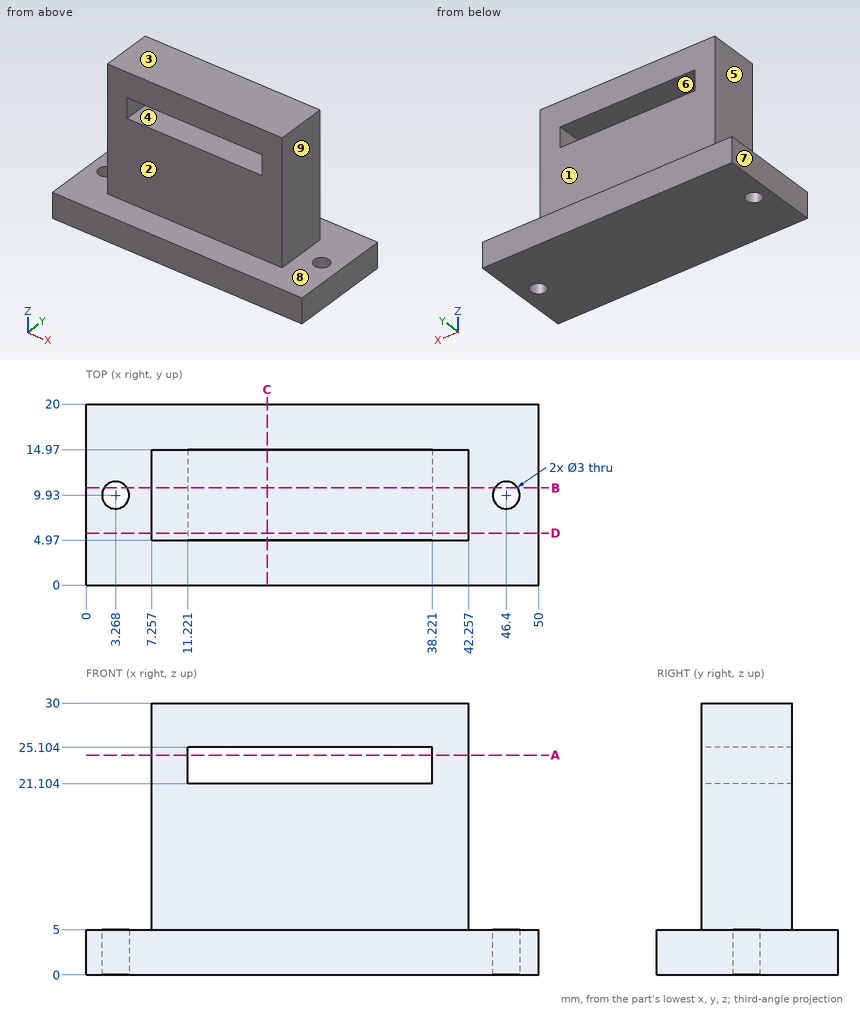
Print and shaded views of the part. All mm, measured from the part's lowest x, y and z. A direction names the side the tool comes from. Round coordinates to 2 decimals unless told otherwise and drop trailing zeros. Write each loop counter-clockwise with the first axis right and the second up, starting at its lowest first coordinate (ties: lowest second). Pieces come first, ordered by that corner, then holes. Notation, with made-up numbers: (75, -22) -> (99, -22) arc R6 ccw to (99, -15) -> close; hole circle Ø5 at (-15.75, -37). An arc over 180 degrees is marked (long way). Answer in a Markdown table with one row per item. Add a question column.
Item 1: Which spindle directions (+Z, -Z, +X, -X, +Y, -Y) get a long thin tool onto all of the face, cutting with end or side? Do the marked faces 1, 2, 3, 4 and 5. Say none if no direction does.
Item 2: Saw through at A-A, the plane z = 24.25. Write the cut outline in (x, y), then the cut area to 3 significant figures.
Item 3: Saw through at D-D, the plane y = 5.75. Write the cut outline in (x, z) (1 decimal), then the cut area to 3 significant figures.
Item 4: Mould opens along X. For the marked faces 6, 7, 8 and 9 say: pulls with the +X half, pulls with the -X half, needs draft (parallel to the pull), parting line crosses it, or undercut.
Item 5: Saw through at B-B, the plane y = 10.75. Write the cut outline in (x, z) (1 decimal), then the cut area to 3 significant figures.
Item 6: Saw through at C-C, the plane x = 20. Write the cut outline in (y, z) (1 decimal).
Item 7: Drop flat-ended pins along their axis: pin 1 Ø2 at (y, z) = (8, 19) entering from -X; pin 2 Ø5 at (y, z) = (7.5, 14.5) entering from +X; pin 3 Ø1.5 at (x, y) = (39.5, 4) entering from +Z. Give the stop position or say it passes through.
Item 8: Drill centre lines: line 1 (Z direction, x = 13, y = 7.25) (1 decimal); line 2 (Y direction, x = 35, z = 27.75); line 3 (Z direction, x = 20, y = 3.5). Where is each one in solid material? Low to high. Write a range as from..to.
Findings below:
| question | item | result |
|---|---|---|
| 1 | face 1 | +Z, +X, -X, +Y |
| 1 | face 2 | +Z, +X, -X, -Y |
| 1 | face 3 | +Z, +X, -X, +Y, -Y |
| 1 | face 4 | +Y, -Y |
| 1 | face 5 | +Z, -X, +Y, -Y |
| 2 | outline | (7.26, 4.97) -> (11.22, 4.97) -> (11.22, 14.97) -> (7.26, 14.97) -> close; (38.22, 4.97) -> (42.26, 4.97) -> (42.26, 14.97) -> (38.22, 14.97) -> close |
| 2 | area | 80.0 mm^2 |
| 3 | outline | (0, 0) -> (50, 0) -> (50, 5) -> (42.3, 5) -> (42.3, 30) -> (7.3, 30) -> (7.3, 5) -> (0, 5) -> close; hole (11.2, 21.1) -> (38.2, 21.1) -> (38.2, 25.1) -> (11.2, 25.1) -> close |
| 3 | area | 1,020 mm^2 |
| 4 | face 6 | undercut |
| 4 | face 7 | pulls with the -X half |
| 4 | face 8 | needs draft |
| 4 | face 9 | pulls with the +X half |
| 5 | outline | (0, 0) -> (2, 0) -> (2, 5) -> (0, 5) -> close; (4.5, 0) -> (45.1, 0) -> (45.1, 5) -> (42.3, 5) -> (42.3, 30) -> (7.3, 30) -> (7.3, 5) -> (4.5, 5) -> close; (47.7, 0) -> (50, 0) -> (50, 5) -> (47.7, 5) -> close; hole (11.2, 21.1) -> (38.2, 21.1) -> (38.2, 25.1) -> (11.2, 25.1) -> close |
| 5 | area | 992 mm^2 |
| 6 | outline | (0, 0) -> (20, 0) -> (20, 5) -> (15, 5) -> (15, 21.1) -> (5, 21.1) -> (5, 5) -> (0, 5) -> close; (5, 25.1) -> (15, 25.1) -> (15, 30) -> (5, 30) -> close |
| 7 | pin 1 | stops at x = 7.26 |
| 7 | pin 2 | stops at x = 42.26 |
| 7 | pin 3 | stops at z = 5 |
| 8 | line 1 | z = 0..21.1, 25.1..30 |
| 8 | line 2 | y = 4.97..14.97 |
| 8 | line 3 | z = 0..5 |
